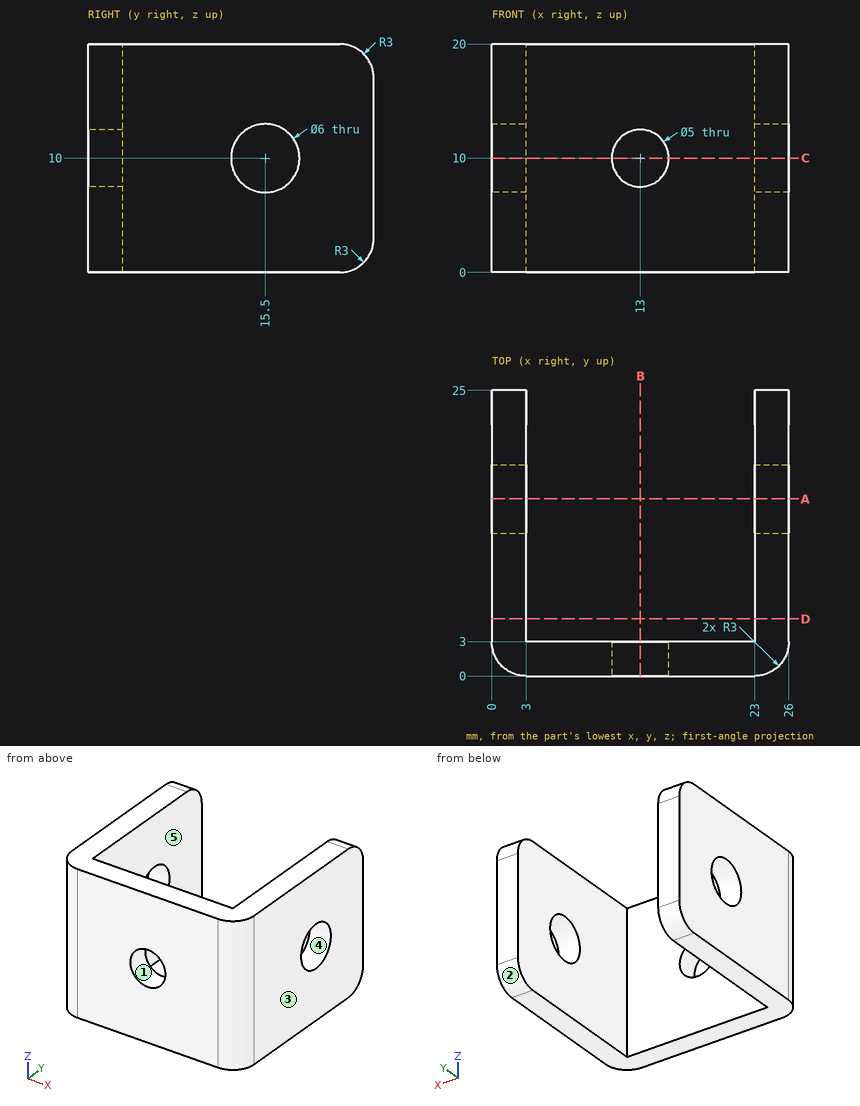
Geometry check sheet. Reference: drawing and pictorial views, mm from the part's lowest x, y, z. A direction names the side the tool comes from. Give positions to 0.01 mm unless a question says otherwise; leave off trailing zeros. Loops run counter-clockwise (first coordinate to the right, second up) from the corner with the lowest first, then second, coordinate; pieces in that order, holes last. Notation, with made-up numbers: M 4.25,-13.5 L 35.25,-13.5 A22 ccw 35.25,11.5 Z; hole C 12.25,-38 d1. An arc over 180 degrees is marked long. One line per question, with ' | ' between items.
Item 1: Tool access check on the marked faces 4 and 5. Record the directions out of +Z, -Z, +X, -X, +Y, -Y that give a thin tool (end or side, any length) a straight path to the whole face; none if there is none.
Completed:
face 4: +X, -X | face 5: +Z, -Z, +Y
Item 2: Section check D-D, the plane y = 5. Record the cut outline in (x, z).
Completed:
outline: M 0,0 L 3,0 L 3,20 L 0,20 Z; M 23,0 L 26,0 L 26,20 L 23,20 Z
Item 3: Section check A-A, the plane y = 15.5. Record the cut outline in (x, z), plus the area to 3 significant figures.
Completed:
outline: M 0,0 L 3,0 L 3,7 L 0,7 Z; M 0,13 L 3,13 L 3,20 L 0,20 Z; M 23,0 L 26,0 L 26,7 L 23,7 Z; M 23,13 L 26,13 L 26,20 L 23,20 Z | area: 84.0 mm^2
Item 4: Depth check by flat-ended pin: P1, Ø2, axis at x = 13.5, z = 14.5, coming from the +Y side. Enter the tip coordinate at first touch or a pass-through.
Completed:
P1: stops at y = 3
Item 5: Section check B-B, the plane x = 13. Record the cut outline in (y, z), plus the area to 3 significant figures.
Completed:
outline: M 0,0 L 3,0 L 3,7.5 L 0,7.5 Z; M 0,12.5 L 3,12.5 L 3,20 L 0,20 Z | area: 45.0 mm^2
Item 6: Section check C-C, the plane z = 10. Record the cut outline in (x, y).
Completed:
outline: M 0,3 A3 ccw 3,0 L 10.5,0 L 10.5,3 L 3,3 L 3,12.5 L 0,12.5 Z; M 0,18.5 L 3,18.5 L 3,25 L 0,25 Z; M 15.5,0 L 23,0 A3 ccw 26,3 L 26,12.5 L 23,12.5 L 23,3 L 15.5,3 Z; M 23,18.5 L 26,18.5 L 26,25 L 23,25 Z
Item 7: Draft check along Z on the marked faces 1, 2 and 3. Enter one of: +Z half, -Z half, draft (parallel to the pull), parting line (faces both ways), or undercut.
Completed:
face 1: undercut | face 2: -Z half | face 3: draft
Item 8: Thickness scan on line 1 (X direction, y = 20.5, z = 15); line 2 (Z direction, x = 13, y = 1.6); line 3 (Y direction, x = 1, z = 10). Record the ranges inside material, lowest first. Write a range as [from, to].
Completed:
line 1: x = [0, 3], [23, 26] | line 2: z = [0, 7.5], [12.5, 20] | line 3: y = [0.76, 12.5], [18.5, 25]
